Verification items for the finished model (mm, model axes). Coordinates: 2 decimals unless noted, no trailing zeros. Loops run counter-clockwise (first coordinate to the right, second up) from the corner with the lowest first, then second, coordinate; pieces in that order, holes last. Notation, with made-up numbers: (46.25, 78) -> (51.25, 78) arc R27 ccw to (51.25, 102) -> close; hole circle Ø9 at (19.5, -33). An arc over 180 degrees is marked (long way). Answer as a JSON object with one key per item and string values. Group by question number.
Q1. Gauge pin test, flat ends, axial feed: pin 1 Ø1 at (y, z) = (0.5, -7) entering from -X; pin 2 Ø3 at (x, y) = (8, 1.5) entering from +Z; pin 3 Ø1 at (y, z) = (3.5, 5) entering from -X. Record the tip position at first contact, or that the pin passes through.
Q2. Cross-section at A-A on y = 2.6. Record the boundary of the cut face in (x, z), and give its area (3 significant figures).
Q3. Scan lines: L1, parallel to Y at x = -4.75, z = -8.5; L2, parallel to X at y = 3.2, z = -6.25; L3, parallel to Z at x = -7.25, y = 4.1. Record each from-to range of solid material in increasing order.
```python
from build123d import *

# Parameters (mm, degrees)
SKETCH1_R           = 10
BOSS_EXTRUDE1_DEPTH = 5
CUT_EXTRUDE1_START  = -0.762
SKETCH2_R           = 10
SKETCH2_R_2         = 9.492
CUT_EXTRUDE1_DEPTH  = 0.762
FILLET3_R           = 1.27
FILLET2_R           = 0.127


with BuildPart() as part:
    # Sketch1 → Boss-Extrude1 (new body)
    with BuildSketch(Plane(origin=(0, 0, 0), x_dir=(1, 0, 0), z_dir=(0, 1, 0))):
        with Locations(Location((0, 0, 0), (0, 0, 270))):
            Circle(SKETCH1_R)
    extrude(amount=BOSS_EXTRUDE1_DEPTH)

    # Sketch2 → Cut-Extrude1 (cut)
    with BuildSketch(Plane(origin=(0, 5, 0), x_dir=(1, 0, 0), z_dir=(0, 1, 0)).offset(CUT_EXTRUDE1_START)):
        with Locations(Location((0, 0, 0), (0, 0, 270))):
            Circle(SKETCH2_R)
        with Locations(Location((0, 0, 0), (0, 0, 270))):
            Circle(SKETCH2_R_2, mode=Mode.SUBTRACT)
    extrude(amount=CUT_EXTRUDE1_DEPTH, mode=Mode.SUBTRACT)

    # Fillet3
    # the kernel refuses this fillet: 1.27 mm, written as the material it takes off along each edge
    with BuildSketch(Plane(origin=(0, 5, 0), x_dir=(0, 0, 1), z_dir=(-1, 0, 0))) as fillet3_piece_1:
        with BuildLine():
            CenterArc((8.328025773, -1.27), FILLET3_R, 23.578178478, 66.421821522)
            Line((8.328025773, 0), (8.328025773, 0.0254))
            Line((8.328025773, 0.0254), (9.492, 0.0254))
            Line((9.492, 0.0254), (9.5174, 0))
            ThreePointArc((9.5174, 0), (9.5174, -0.381), (9.515279485, -0.75184))
            Line((9.515279485, -0.75184), (9.492, -0.762))
        make_face()
    revolve(axis=Axis((0, 5, 0), (0, 1, 0)), mode=Mode.SUBTRACT)

    # Fillet2
    fillet2_edges = [part.edges().sort_by_distance(p)[0] for p in [
        (0, 0, -10),
        (0, 4.238, -10),
    ]]
    fillet(fillet2_edges, radius=FILLET2_R)


solid = part.part
```
Computed values:
{
 "1": {"pin 1": "stops at x = -7.6", "pin 2": "stops at z = 7.6", "pin 3": "stops at x = -8.93"},
 "2": {"outline": "circle Ø20 at (0, 0)", "area": "314 mm²"},
 "3": {"L1": "y = 0 to 4.24", "L2": "x = -7.81 to 7.81", "L3": "z = -6.89 to 6.89"}
}
